Verification items for the finished model (mm, model axes). Face numbers are marked on the shaded views. Coordinates: 2 decimals unless noted, no trailing zeros. Answer as a JSON object with one key per item and string values. Group by question number.
Q1. Gauge pin test, flat ends, axial feed: pin 1 Ø5 at (x, z) = (17, 25) entering from -Y (3 decimals); pin 2 Ø4 at (y, z) = (22, 6.5) entering from +X; pin 3 Ø1 at (y, z) = (-18.5, 5) entering from +X; pin 4 Ø8 at (y, z) = (8.5, 41.5) entering from -X. Record the tip position at first contact, or that the pin passes through.
Q2. Release check for a two-part mould opening along X. For the marked faces 1 and 2 record: released by +X, released by -X, zero draft, split by the parting line, or undercut.
Q3. Scan lines: L1, parallel to Z at x = 9, y = 21.5; L2, parallel to X at y = 13, z = 27; L3, parallel to X at y = 34.5, z = 19.5. Record each from-to range of solid material in increasing order.
```python
from build123d import *

# Parameters (mm, degrees)
F0_W        = 111.22
F0_H        = 71.63
F2_W        = 121.14
F2_H        = 85.07
F4_R        = 5
F6_W        = 123.14
F6_H        = 87.07
F7_DEPTH    = 6
F8_T1_DEPTH = 154.335608958
F8_T3_DEPTH = 118.265608958
F10_W       = 101.22
F10_H       = 61.63
F11_DEPTH   = 1
F12_R       = 5


# Not quite as in the source:
# - a fillet or chamfer that OpenCascade refuses, or shapes differently, is made with other operations: its cross-section is extruded or revolved along the edge and cut away or added


with BuildPart() as f3:
    # F0 (on Top) → F3 section 0
    with BuildSketch(Plane.XY):
        Rectangle(F0_W, F0_H)
    # F2 (on offset) → F3 section 1
    with BuildSketch(Plane.XY.offset(42)):
        Rectangle(F2_W, F2_H)
    loft()

    # F4
    f4_edges = [f3.edges().sort_by_distance(p)[0] for p in [
        (-58.09, -39.175, 21),
        (0, -35.815, 0),
        (58.09, -39.175, 21),
        (55.61, 0, 0),
        (58.09, 39.175, 21),
        (0, 35.815, 0),
        (-58.09, 39.175, 21),
        (-55.61, 0, 0),
    ]]
    fillet(f4_edges, radius=F4_R)

    # F6 (on offset) → F7 (join)
    with BuildSketch(Plane.XY.offset(42)):
        Rectangle(F6_W, F6_H)
    extrude(amount=F7_DEPTH)

    # F8: chamfer of 6 x 0.5249319812 on 4 edges, made by hand

    # F8_s2 → F8_t1 (cut)
    with BuildSketch(Plane.YZ.offset(-77.167804479)):
        Polygon((-43.535, 42), (-43.0100680188, 48), (-43.535, 48), align=None)
        Polygon((43.535, 42), (43.0100680188, 48), (43.535, 48), align=None)
    extrude(amount=F8_T1_DEPTH, mode=Mode.SUBTRACT)

    # F8_s4 → F8_t3 (cut)
    with BuildSketch(Plane.XZ.offset(-59.132804479)):
        Polygon((-61.0450680188, 48), (-61.57, 42), (-61.57, 48), align=None)
        Polygon((61.57, 42), (61.0450680188, 48), (61.57, 48), align=None)
    extrude(amount=F8_T3_DEPTH, mode=Mode.SUBTRACT)

    # F10 (on offset) → F11 (cut)
    with BuildSketch(Plane.XY.offset(48)):
        Rectangle(F10_W, F10_H)
    extrude(amount=-F11_DEPTH, mode=Mode.SUBTRACT)

    # F12
    f12_edges = [f3.edges().sort_by_distance(p)[0] for p in [
        (-61.307534, -43.272534, 45),
        (61.307534, -43.272534, 45),
        (61.307534, 43.272534, 45),
        (-61.307534, 43.272534, 45),
    ]]
    fillet(f12_edges, radius=F12_R)


solid = f3.part
```
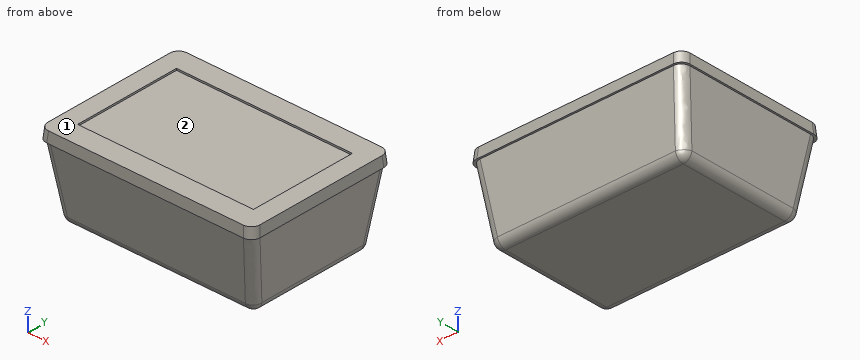
Computed values:
{
 "1": {"pin 1": "stops at y = -40.215", "pin 2": "stops at x = 56.61", "pin 3": "stops at x = 56.26", "pin 4": "stops at x = -61.57"},
 "2": {"face 1": "zero draft", "face 2": "undercut"},
 "3": {"L1": "z = 0 to 47", "L2": "x = -58.8 to 58.8", "L3": "x = -57.88 to 57.88"}
}
